from build123d import *

# Parameters (mm, degrees)
F0_W     = 9.9
F0_H     = 12.5
F0_R     = 2.25
F1_DEPTH = 4


with BuildPart() as f1:
    # F0 (on Right) → F1 (new body)
    with BuildSketch(Plane.YZ):
        Rectangle(F0_W, F0_H)
        Circle(F0_R, mode=Mode.SUBTRACT)
    extrude(amount=-F1_DEPTH)


solid = f1.part
Input: part model. Units: mm. Frame: model coordinates. Coordinates: 2 decimals unless noted, no trailing zeros. Loops run counter-clockwise (first coordinate to the right, second up) from the corner with the lowest first, then second, coordinate; pieces in that order, holes last.
(1) Section A-A on y = 0. Return the cut outline in (x, z), then the cut area to 3 significant figures.
(2) Section B-B on x = -0.4. Return the cut outline in (y, z).
(3) First-contact query: pin 1 Ø1 at (y, z) = (-1, -5) entering from +X. Flat tip, straight axial feed; report the tip coordinate or a pass-through.
(4) Section C-C on z = -1.75. Return the cut outline in (x, y).
(5) Material intervals for probe 1 along Z at (x, y) = (-2.4, 0); probe 2 along Y at (x, z) = (-0.8, 1.25); probe 3 along Y at (x, z) = (-2.8, -2), sorted ascending.
Data:
1. outline: (-4, -6.25) - (0, -6.25) - (0, -2.25) - (-4, -2.25) - close; (-4, 2.25) - (0, 2.25) - (0, 6.25) - (-4, 6.25) - close
1. area: 32.0 mm2
2. outline: (-4.95, -6.25) - (4.95, -6.25) - (4.95, 6.25) - (-4.95, 6.25) - close; hole circle Ø4.5 at (0, 0)
3. pin 1: stops at x = 0
4. outline: (-4, -4.95) - (0, -4.95) - (0, -1.41) - (-4, -1.41) - close; (-4, 1.41) - (0, 1.41) - (0, 4.95) - (-4, 4.95) - close
5. probe 1: z = -6.25 to -2.25, 2.25 to 6.25
5. probe 2: y = -4.95 to -1.87, 1.87 to 4.95
5. probe 3: y = -4.95 to -1.03, 1.03 to 4.95
